```python
from build123d import *

# Parameters (mm, degrees)
SKETCH6_W           = 128
SKETCH6_H           = 73
BOSS_EXTRUDE1_DEPTH = 4
SKETCH7_W           = 128
SKETCH7_H           = 73
SKETCH7_W_2         = 120
SKETCH7_H_2         = 65
BOSS_EXTRUDE2_DEPTH = 41
BOSS_EXTRUDE4_DEPTH = 34
CUT_EXTRUDE1_REACH  = 75
SKETCH10_R          = 10.16
CUT_EXTRUDE2_REACH  = 130


with BuildPart() as part:
    # Sketch6 → Boss-Extrude1 (new body)
    with BuildSketch(Plane(origin=(0, 0, 0), x_dir=(1, 0, 0), z_dir=(0, 1, 0))):
        Rectangle(SKETCH6_W, SKETCH6_H)
    extrude(amount=-BOSS_EXTRUDE1_DEPTH)

    # Sketch7 → Boss-Extrude2 (add)
    with BuildSketch(Plane.XZ.offset(4)):
        Rectangle(SKETCH7_W, SKETCH7_H)
        Rectangle(SKETCH7_W_2, SKETCH7_H_2, mode=Mode.SUBTRACT)
    extrude(amount=BOSS_EXTRUDE2_DEPTH)

    # Sketch9 → Boss-Extrude4 (add)
    with BuildSketch(Plane.XZ.offset(4)):
        Polygon((-5, 32.5), (-5, -32.5), (-18.5, -32.5), (-18.5, -21.3), (-15, -21.3), (-15, -26.3), (-11, -26.3), (-11, 26.3), (-15, 26.3), (-15, 21.3), (-18.5, 21.3), (-18.5, 32.5), align=None)
    extrude(amount=BOSS_EXTRUDE4_DEPTH)

    # Sketch10 → Cut-Extrude1 (cut, up to next)
    with BuildSketch(Plane(origin=(0, 0, -36.5), x_dir=(-1, 0, 0), z_dir=(0, 0, -1)), mode=Mode.PRIVATE) as cut_extrude1_sk1:
        with Locations((44, -25)):
            Circle(SKETCH10_R)
    cut_extrude1_tool1 = extrude(cut_extrude1_sk1.sketch, amount=-CUT_EXTRUDE1_REACH, mode=Mode.PRIVATE) & part.part
    add(cut_extrude1_tool1.solids().sort_by_distance((-44, -25, -36.5))[0], mode=Mode.SUBTRACT)

    # Sketch13 → Cut-Extrude2 (cut, up to next)
    with BuildSketch(Plane.ZY.offset(64), mode=Mode.PRIVATE) as cut_extrude2_sk1:
        with BuildLine():
            Line((-12, -21), (12, -21))
            ThreePointArc((12, -21), (16, -25), (12, -29))
            Line((12, -29), (-12, -29))
            ThreePointArc((-12, -29), (-16, -25), (-12, -21))
        make_face()
    cut_extrude2_tool1 = extrude(cut_extrude2_sk1.sketch, amount=-CUT_EXTRUDE2_REACH, mode=Mode.PRIVATE) & part.part
    add(cut_extrude2_tool1.solids().sort_by_distance((-64, -25, 0))[0], mode=Mode.SUBTRACT)


solid = part.part
```
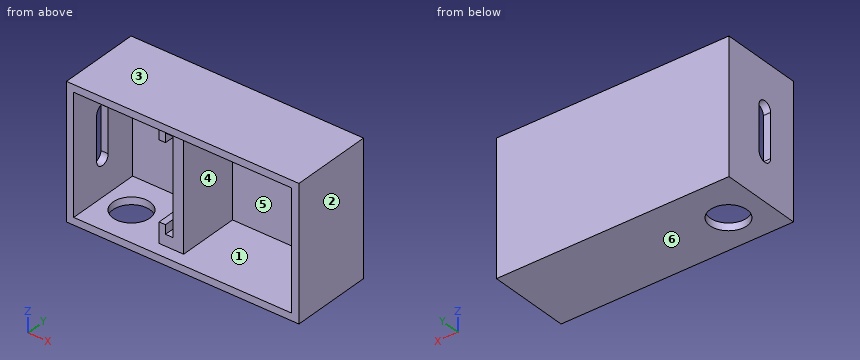
Geometry: final body of the model. Coordinates: model frame, mm. Face numbers are marked on the shaded views. A direction names the side the tool comes from. Give positions to 0.01 mm unless a question says otherwise; leave off trailing zeros. Loops run counter-clockwise (first coordinate to the right, second up) from the corner with the lowest first, then second, coordinate; pieces in that order, holes last. Notation, with made-up numbers: (64, 41.5) -> (92, 41.5) arc R6 cw to (92, 52.5) -> close; hole circle Ø9 at (52, 49.25). An arc over 180 degrees is marked (long way). Return JSON: item names as keys, results as strings.
Item 1: Line query: line 1 (X direction, y = -14, z = 13); line 2 (X direction, y = -26.5, z = 31); line 3 (X direction, y = -42, z = -29). Output: solid intervals per line, ascending.
Filled in:
{"line 1": "-64 to -60, -11 to -5, 60 to 64", "line 2": "-64 to -60, -18.5 to -5, 60 to 64", "line 3": "-64 to -60, 60 to 64"}
Item 2: Access query for the marked faces 5 and 6. Directions: +Z, -Z, +X, -X, +Y, -Y. A direction counts if a zero-diameter tool reaches every point of the face in a straight line with its end or side. Return the directions, or none.
Filled in:
{"face 5": "-Y", "face 6": "-Z, +X, -X, +Y, -Y"}
Item 3: Mould query, pull axis Z, two halves, no side actions, for the marked faces 1, 2, 3 and 4. Classes: released by +Z, released by -Z, zero draft, split by the parting line, or undercut.
Filled in:
{"face 1": "undercut", "face 2": "zero draft", "face 3": "released by +Z", "face 4": "undercut"}
Item 4: Section B-B, the plane x = -44. Output: boundary loops of the cut face in (y, z).
Filled in:
{"outline": "(-45, -36.5) -> (-35.16, -36.5) -> (-35.16, -32.5) -> (-45, -32.5) -> close; (-45, 32.5) -> (-4, 32.5) -> (-4, -32.5) -> (-14.84, -32.5) -> (-14.84, -36.5) -> (0, -36.5) -> (0, 36.5) -> (-45, 36.5) -> close"}
Item 5: Pin query (flat end, axial travel): P1, Ø18.5, axis at x = -44, y = -25, coming from the -Z side; P2, Ø24.5, axis at x = -39, z = -4.5, coming from the -Y side. Return the tip coordinate at first contact, or that it passes through.
Filled in:
{"P1": "z = 32.5", "P2": "y = -4"}
Item 6: Section D-D, the plane y = -30.5. Output: boundary loops of the cut face in (x, z).
Filled in:
{"outline": "(-64, -36.5) -> (-52.54, -36.5) -> (-52.54, -32.5) -> (-60, -32.5) -> (-60, 32.5) -> (-18.5, 32.5) -> (-18.5, 21.3) -> (-15, 21.3) -> (-15, 26.3) -> (-11, 26.3) -> (-11, -26.3) -> (-15, -26.3) -> (-15, -21.3) -> (-18.5, -21.3) -> (-18.5, -32.5) -> (-35.46, -32.5) -> (-35.46, -36.5) -> (64, -36.5) -> (64, 36.5) -> (-64, 36.5) -> close; hole (-5, -32.5) -> (60, -32.5) -> (60, 32.5) -> (-5, 32.5) -> close"}
Item 7: Section A-A, the plane y = -25. Output: boundary loops of the cut face in (x, z).
Filled in:
{"outline": "(-64, -36.5) -> (-54.16, -36.5) -> (-54.16, -32.5) -> (-60, -32.5) -> (-60, -16) -> (-64, -16) -> close; (-64, 16) -> (-60, 16) -> (-60, 32.5) -> (-18.5, 32.5) -> (-18.5, 21.3) -> (-15, 21.3) -> (-15, 26.3) -> (-11, 26.3) -> (-11, -26.3) -> (-15, -26.3) -> (-15, -21.3) -> (-18.5, -21.3) -> (-18.5, -32.5) -> (-33.84, -32.5) -> (-33.84, -36.5) -> (64, -36.5) -> (64, 36.5) -> (-64, 36.5) -> close; hole (-5, -32.5) -> (60, -32.5) -> (60, 32.5) -> (-5, 32.5) -> close"}
Item 8: Section C-C, the plane x = -2. Output: boundary loops of the cut face in (y, z), plus the area to 3 significant figures.
Filled in:
{"outline": "(-45, -36.5) -> (0, -36.5) -> (0, 36.5) -> (-45, 36.5) -> (-45, 32.5) -> (-4, 32.5) -> (-4, -32.5) -> (-45, -32.5) -> close", "area": "620 mm^2"}
